Autodesk Inventor part; units mm, degrees
ref_plane "YZ Plane" through (0, 0, 0) normal (1, 0, 0) x (0, 1, 0)
ref_plane "XZ Plane" through (0, 0, 0) normal (0, 1, 0) x (-1, 0, 0)
ref_plane "XY Plane" through (0, 0, 0) normal (0, 0, 1) x (1, 0, 0)
sketch "Sketch1" plane through (0, 0, 0) normal (1, 0, 0) x (0, 1, 0)
  line L0 (0, 0) -> (25.4, 0)
  line L1 (25.4, 0) -> (25.4, -3.175)
  line L2 (25.4, -3.175) -> (3.175, -3.175)
  line L3 (3.175, -3.175) -> (3.175, -25.4)
  line L4 (3.175, -25.4) -> (0, -25.4)
  line L5 (0, -25.4) -> (0, 0)
  dimension "d0" = 25.4
  dimension "d1" = 3.175
  dimension "d2" = 22.225
  dimension "d3" = 22.225
  dimension "d4" = 3.175
extrude "Extrusion1" add sketch "Sketch1" along normal blind 1022.1976
sketch "Sketch3" plane through (0, 0, 0) normal (0, 0, 1) x (1, 0, 0)
  line L0 (1022.1976, 0) -> (1022.1976, 25.4)
  line L1 (1022.1976, 25.4) -> (996.7976, 25.4)
  line L2 (996.7976, 25.4) -> (1022.1976, 0)
  line L3 (0, 25.4) -> (0, 0)
  line L4 (0, 0) -> (0, 25.4)
  line L5 (0, 0) -> (25.4, 0)
  line L6 (25.4, 0) -> (0, 25.4)
  dimension "d11" = 25.4
  dimension "d12" = 25.4
  dimension "d13" = 45
extrude "Extrusion3" cut sketch "Sketch3" against normal blind 1022.1976
properties part number "Brace Back 45"
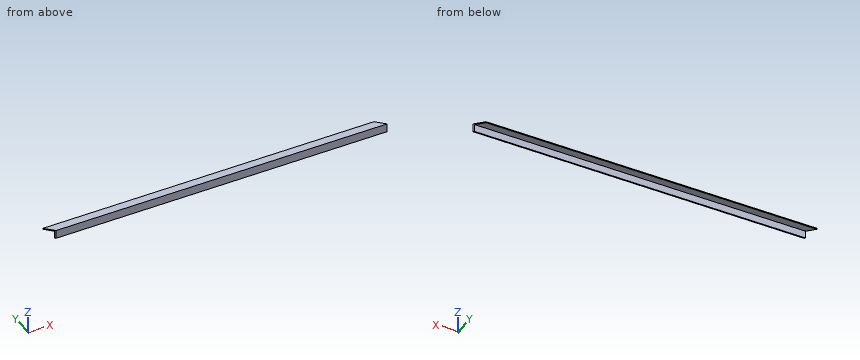
Here's how the part is built. I have some questions about the finished solid (model axes, mm). Coordinates: 2 decimals unless noted, no trailing zeros. Loops run counter-clockwise (first coordinate to the right, second up) from the corner with the lowest first, then second, coordinate; pieces in that order, holes last. Notation, with made-up numbers: (-11, 43) - (46, 43) arc R10 cw to (46, 48) - close; hole circle Ø7 at (2.25, 18.5). An arc over 180 degrees is marked (long way). Return JSON: item names as keys, results as strings. Group by question number.
Item 1: If we section it at A-A on x = 810: Write out the boundary of the cut face in (y, z) (3 decimals), and give its area (3 significant figures).
Item 2: I need wall thicknesses on line 1 (Z direction, x = 955.5, y = 6.5) (3 decimals); line 2 (Y direction, x = 78, z = -23.25) (3 decimals); line 3 (X direction, y = 18, z = -2.75). Which ranges of each line are inside material? Lowest first, please. Write a range as from..to.
Item 3: If we section it at C-C on y = 9: Write out the boundary of the cut face in (x, z) (3 decimals), and give its area (3 significant figures).
Item 4: If we section it at B-B on z = -11.5: Write out the boundary of the cut face in (x, y) (3 decimals).
Item 5: Will these pins go through, and if not, where does the flat tip stop? P1, Ø10, axis at x = 636.5, z = -14.5, coming from the +Y side (3 decimals); P2, Ø8, axis at y = 4.5, z = -8.5, coming from the -X side (3 decimals); P3, Ø5, axis at x = 616.5, y = 13.5, coming from the -Z side (3 decimals).
Calculated:
{
 "1": {"outline": "(0, -25.4) - (3.175, -25.4) - (3.175, -3.175) - (25.4, -3.175) - (25.4, 0) - (0, 0) - close", "area": "151 mm^2"},
 "2": {"line 1": "z = -3.175..0", "line 2": "y = 0..3.175", "line 3": "x = 7.4..1004.2"},
 "3": {"outline": "(16.4, -3.175) - (1013.198, -3.175) - (1013.198, 0) - (16.4, 0) - close", "area": "3,160 mm^2"},
 "4": {"outline": "(22.225, 3.175) - (25.4, 0) - (1022.198, 0) - (1019.023, 3.175) - close"},
 "5": {"P1": "stops at y = 3.175", "P2": "stops at x = 22.225", "P3": "stops at z = -3.175"}
}
